```python
from build123d import *

# Parameters (mm, degrees)
F0_R     = 40.1789827743
F1_DEPTH = 5.08
F2_R     = 19.6940122024
F3_DEPTH = 2.54
F4_R     = 5.07999


# Not quite as in the source:
# - a fillet or chamfer that OpenCascade refuses, or shapes differently, is made with other operations: its cross-section is extruded or revolved along the edge and cut away or added
# - a fillet or chamfer is up to 0.001 mm smaller than in the source, because OpenCascade refuses the exact size


with BuildPart() as f1:
    # F0 (on Front) → F1 (new body)
    with BuildSketch(Plane.XZ):
        Circle(F0_R)
    extrude(amount=F1_DEPTH)

    # F2 (on face) → F3 (join)
    with BuildSketch(Plane.XZ.offset(5.08)):
        with Locations((5.5896993726, 0)):
            Circle(F2_R)
    extrude(amount=F3_DEPTH)

    # F4 (radius 5.08 in the source; OpenCascade refuses exactly that, so slightly less here)
    f4_edges = [f1.edges().sort_by_distance(p)[0] for p in [
        (-40.178983, -5.08, 0),
    ]]
    fillet(f4_edges, radius=F4_R)

    # F5: fillet of radius 5.08 on 1 edges, made by hand

    # F5_s1 → F5_t2 (revolve, cut)
    with BuildSketch(Plane.XY):
        with BuildLine():
            ThreePointArc((25.283711575, -5.08), (23.4243025238, -6.9394090512), (20.8843025238, -7.62))
            Line((20.8843025238, -7.62), (25.283711575, -7.62))
            Line((25.283711575, -7.62), (25.283711575, -5.08))
        make_face()
    revolve(axis=Axis((5.5896993726, -7.62, 0), (0, -1, 0)), mode=Mode.SUBTRACT)


solid = f1.part
```
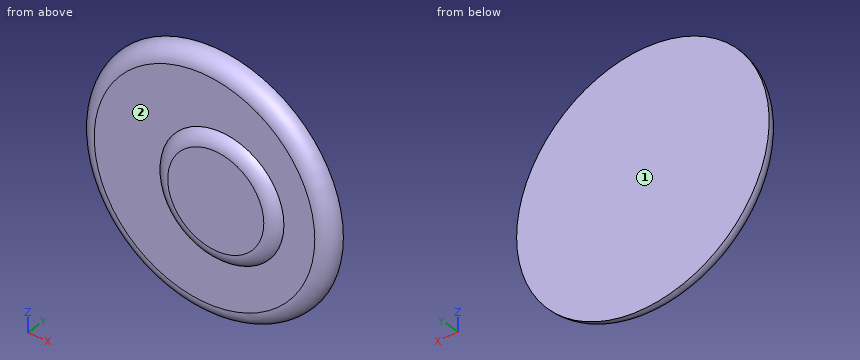
Model file for the job. Use its own axes, mm. Face numbers are marked on the shaded views. A direction names the side the tool comes from. Round coordinates to 2 decimals unless told otherwise and drop trailing zeros. Order: outer loops, then holes, each group sorted by start corner. A loop starts at its lowest first (then second) coordinate and runs counter-clockwise, first axis right, second up. Notation, with made-up numbers: (88.5, 56.5) -> (103.5, 56.5) arc R29 ccw to (103.5, 79.5) -> close; hole circle Ø8 at (-28, 70). An arc over 180 degrees is marked (long way). Use one line per item in the form item = value.
Item 1: Flat gauge pins, fed straight in: pin 1 Ø4 at (x, z) = (1.5, 17.5) entering from -Y; pin 2 Ø4 at (x, y) = (-0.5, -6.5) entering from +Z; pin 3 Ø4 at (x, y) = (26, -4) entering from +Z. Where does each tip first touch, or does it go through?
Returned:
pin_1 = -7.57
pin_2 = 37.45
pin_3 = 30.88
Item 2: Drill centre lines: line 1 (Y direction, x = -15.5, z = -17); line 2 (X direction, y = -6, z = 4); line 3 (Z direction, x = 7, y = -4.25). Where is each one in solid material? Low to high.
Returned:
line_1 = -5.08 to 0
line_2 = -13 to 24.18
line_3 = -37.23 to 37.23
Item 3: Cut at B-B, the plane y = -6.5. Write the cut outline in (x, z).
Returned:
outline = circle Ø36.95 at (5.59, 0)
Item 4: Tool access for the marked faces 1 and 2: list every direction of +Z, -Z, +X, -X, +Y, -Y with a clear straight run to the whole face (end or side of a thin tool).
Returned:
face_1 = +Z, -Z, +X, -X, +Y
face_2 = -Y
Item 5: Cut at C-C, the plane y = -1. Write the cut outline in (x, z).
Returned:
outline = circle Ø80.16 at (0, 0)
